```python
from build123d import *

# Parameters (mm, degrees)
SKETCH_1_W               = 50
SKETCH_1_H               = 20
SKETCH_1_W_2             = 150
SKETCH_1_H_2             = 80
EXTRUDE_3_DEPTH          = 80
SKETCH_3_W               = 80
SKETCH_3_H               = 20
EXTRUDE_4_DEPTH          = 50
CUT_EXTRUDE_1_DEPTH      = 181.277563773
CUT_EXTRUDE_1_DEPTH_BACK = 50
SKETCH_5_W               = 50
SKETCH_5_H               = 80
CUT_EXTRUDE_2_DEPTH      = 30
SKETCH_6_W               = 60
SKETCH_6_H               = 15
CUT_EXTRUDE_3_DEPTH      = 15


with BuildPart() as part:
    # Эскиз1 → Бобышка-Вытянуть3 (new body)
    with BuildSketch(Plane.XY):
        with Locations((75, -90)):
            Rectangle(SKETCH_1_W, SKETCH_1_H)
        with Locations((75, -40)):
            Rectangle(SKETCH_1_W_2, SKETCH_1_H_2)
    extrude(amount=EXTRUDE_3_DEPTH)

    # Эскиз3 → Бобышка-Вытянуть4 (add)
    with BuildSketch(Plane.ZY):
        with Locations((40, -50)):
            Rectangle(SKETCH_3_W, SKETCH_3_H)
    extrude(amount=EXTRUDE_4_DEPTH)

    # Эскиз4 → Вырез-Вытянуть1 (cut, two sides: drawn at the far end of the back side and taken through both)
    with BuildSketch(Plane.XZ.offset(60).offset(-CUT_EXTRUDE_1_DEPTH_BACK)):
        Polygon((-50, 70.981091189), (-50, 68.967879487), (0, 80), (-50, 80), align=None)
    extrude(amount=CUT_EXTRUDE_1_DEPTH + CUT_EXTRUDE_1_DEPTH_BACK, mode=Mode.SUBTRACT)

    # Эскиз5 → Вырез-Вытянуть2 (cut)
    with BuildSketch(Plane(origin=(150, 0, 0), x_dir=(0, 0, -1), z_dir=(1, 0, 0))):
        with Locations((-40, -40)):
            Rectangle(SKETCH_5_W, SKETCH_5_H)
    extrude(amount=-CUT_EXTRUDE_2_DEPTH, mode=Mode.SUBTRACT)

    # Эскиз6 → Вырез-Вытянуть3 (cut)
    with BuildSketch(Plane.XY.offset(80)):
        with Locations((75.739234494, -7.5)):
            Rectangle(SKETCH_6_W, SKETCH_6_H)
    extrude(amount=-CUT_EXTRUDE_3_DEPTH, mode=Mode.SUBTRACT)


solid = part.part
```
The listing builds one solid part. Answer for the finished solid, in the listing's coordinates (mm). A direction names the side the tool comes from. Coordinates: 2 decimals unless noted, no trailing zeros. Write each loop counter-clockwise with the first axis right and the second up, starting at its lowest first coordinate (ties: lowest second). Pieces come first, ordered by that corner, then holes. Notation, with made-up numbers: (0.5, -25) - (54.5, -25) arc R21 ccw to (54.5, 13) - close; hole circle Ø10 at (58, 74.5). An arc over 180 degrees is marked (long way). Return JSON: item names as keys, results as strings. Group by question number.
Q1. The part is cut by section A-A on x = 128. Write down the section's boundary in (y, z), and give its area (3 significant figures).
Q2. For a pull along Z with two mould halves and no side action, classify faces 1 (the flat face through (75, -15, 73)), 2 (the flat face through (-25.35, -49.86, 74.407)), 3 (the flat face through (120, -39, 40)) as +Z half, -Z half, draft (parallel to the pull), parting line (faces both ways), or undercut.
Q3. The part is cut by section D-D on z = 11. Write down the section's boundary in (x, y).
Q4. Find the intervals of material crossed by line 1 along Z through (x, y) = (137, -66); line 2 along Y through (x, z) = (-27.5, 21.5); line 3 along X through (y, z) = (-45, 29.5), in increasing order. Write a range as [from, to].
Q5. Which of the six approach directions +Z, -Z, +X, -X, +Y, -Y give full straight-line access (tool end or side, diameter ignored) to faces 4 (the flat face through (0, -70, 39)), 5 (the flat face through (0, -20, 39)), 6 (the flat face through (135, -41, 65)), 7 (the flat face through (75, -7, 65))?
Q6. The part is cut by section C-C on y = -36. Write down the section's boundary in (x, z), and give its area (3 significant figures).
Q7. The part is cut by section B-B on z = 35. Write down the section's boundary in (x, y).
Q8. Flat-ended cylindrical pins translate along their axes: pin 1 Ø15 at (x, z) = (19.5, 42.5) entering from -Y; pin 2 Ø10 at (y, z) = (-32.5, 23.5) entering from +X; pin 3 Ø10 at (y, z) = (-91.5, 49.5) entering from -X. Find the tip coordinate at first contact, or state that the pin passes through.
Evaluation:
{
 "1": {"outline": "(-80, 0) - (0, 0) - (0, 15) - (-80, 15) - close; (-80, 65) - (0, 65) - (0, 80) - (-80, 80) - close", "area": "2,400 mm2"},
 "2": {"face 1": "draft", "face 2": "+Z half", "face 3": "undercut"},
 "3": {"outline": "(-50, -60) - (0, -60) - (0, -80) - (50, -80) - (50, -100) - (100, -100) - (100, -80) - (150, -80) - (150, 0) - (0, 0) - (0, -40) - (-50, -40) - close"},
 "4": {"line 1": "z = [0, 15], [65, 80]", "line 2": "y = [-60, -40]", "line 3": "x = [-50, 120]"},
 "5": {"face 4": "+Z, -Z, -X, -Y", "face 5": "+Z, -Z, -X, +Y", "face 6": "+X, +Y, -Y", "face 7": "+Z, +Y"},
 "6": {"outline": "(0, 0) - (150, 0) - (150, 15) - (120, 15) - (120, 65) - (150, 65) - (150, 80) - (0, 80) - close", "area": "10,500 mm2"},
 "7": {"outline": "(-50, -60) - (0, -60) - (0, -80) - (50, -80) - (50, -100) - (100, -100) - (100, -80) - (120, -80) - (120, 0) - (0, 0) - (0, -40) - (-50, -40) - close"},
 "8": {"pin 1": "stops at y = -80", "pin 2": "stops at x = 120", "pin 3": "stops at x = 50"}
}
